Source: CAD feature listing. Evaluate the final solid. Frame: model axes, mm. Face numbers are marked on the shaded views. A direction names the side the tool comes from. Give positions to 0.01 mm unless a question says otherwise; leave off trailing zeros. Loops run counter-clockwise (first coordinate to the right, second up) from the corner with the lowest first, then second, coordinate; pieces in that order, holes last. Notation, with made-up numbers: M -3.5,70.5 L 52.5,70.5 A34 cw 52.5,106.5 Z; hole C 14,47 d8. An arc over 180 degrees is marked long. Write item = value, one per line.
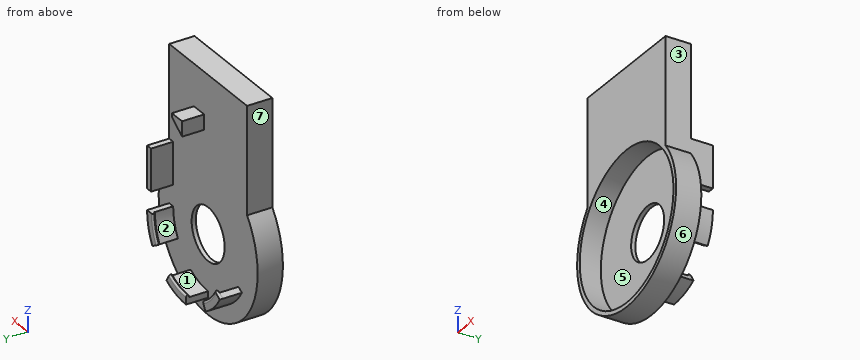
from build123d import *

# Parameters (mm, degrees)
SKETCH1_R           = 37.5
SKETCH1_R_2         = 35.5
BOSS_EXTRUDE1_DEPTH = 10
SKETCH2_R           = 37.5
SKETCH2_R_2         = 12.5
BOSS_EXTRUDE2_DEPTH = 2
BOSS_EXTRUDE3_DEPTH = 9
BOSS_EXTRUDE4_DEPTH = 1.5
FILLET1_R           = 1.27
SKETCH6_W           = 3
SKETCH6_H           = 10.5
BOSS_EXTRUDE5_DEPTH = 30
SKETCH7_W           = 3
SKETCH7_H           = 10
CUT_EXTRUDE1_DEPTH  = 10.5
BOSS_EXTRUDE6_DEPTH = 10.5
BOSS_EXTRUDE8_START = -12
BOSS_EXTRUDE8_DEPTH = 12


with BuildPart() as part:
    # Sketch1 → Boss-Extrude1 (new body)
    with BuildSketch(Plane(origin=(0, 0, 0), x_dir=(1, 0, 0), z_dir=(0, 1, 0))):
        with Locations(Location((0, 0, 0), (0, 0, 270))):
            Circle(SKETCH1_R)
        with Locations(Location((0, 0, 0), (0, 0, 270))):
            Circle(SKETCH1_R_2, mode=Mode.SUBTRACT)
    extrude(amount=BOSS_EXTRUDE1_DEPTH)

    # Sketch2 → Boss-Extrude2 (add)
    with BuildSketch(Plane(origin=(0, 10, 0), x_dir=(1, 0, 0), z_dir=(0, 1, 0))):
        with Locations(Location((0, 0, 0), (0, 0, 270))):
            Circle(SKETCH2_R)
        with Locations(Location((0, 0, 0), (0, 0, 270))):
            Circle(SKETCH2_R_2, mode=Mode.SUBTRACT)
    extrude(amount=BOSS_EXTRUDE2_DEPTH)

    # Sketch4 → Boss-Extrude3 (add)
    with BuildSketch(Plane(origin=(0, 12, 0), x_dir=(1, 0, 0), z_dir=(0, 1, 0))):
        with BuildLine():
            Line((13.25, 22.9496732), (14.75, 25.547749412))
            ThreePointArc((14.75, 25.547749412), (7.635161831, 28.494811876), (0, 29.5))
            Line((0, 29.5), (0, 26.5))
            ThreePointArc((0, 26.5), (6.858704695, 25.597034397), (13.25, 22.9496732))
        make_face()
        with BuildLine():
            ThreePointArc((26.5, 0), (25.597034397, 6.858704695), (22.9496732, 13.25))
            Line((22.9496732, 13.25), (25.547749412, 14.75))
            ThreePointArc((25.547749412, 14.75), (28.494811876, 7.635161831), (29.5, 0))
            Line((29.5, 0), (26.5, 0))
        make_face()
        with BuildLine():
            Line((-13.25, 22.9496732), (-14.75, 25.547749412))
            ThreePointArc((-14.75, 25.547749412), (-20.859650045, 20.859650045), (-25.547749412, 14.75))
            Line((-25.547749412, 14.75), (-22.9496732, 13.25))
            ThreePointArc((-22.9496732, 13.25), (-18.738329701, 18.738329701), (-13.25, 22.9496732))
        make_face()
    extrude(amount=BOSS_EXTRUDE3_DEPTH)

    # Sketch5 → Boss-Extrude4 (add)
    with BuildSketch(Plane(origin=(0, 21, 0), x_dir=(1, 0, 0), z_dir=(0, 1, 0))):
        with BuildLine():
            Line((-12.5, 21.650635095), (-14.75, 25.547749412))
            ThreePointArc((-14.75, 25.547749412), (-20.859650045, 20.859650045), (-25.547749412, 14.75))
            Line((-25.547749412, 14.75), (-21.650635095, 12.5))
            ThreePointArc((-21.650635095, 12.5), (-17.67766953, 17.67766953), (-12.5, 21.650635095))
        make_face()
        with BuildLine():
            ThreePointArc((0, 26.5), (6.858704695, 25.597034397), (13.25, 22.9496732))
            Line((13.25, 22.9496732), (14.75, 25.547749412))
            ThreePointArc((14.75, 25.547749412), (7.635161831, 28.494811876), (0, 29.5))
            Line((0, 29.5), (0, 26.5))
        make_face()
        with BuildLine():
            Line((0, 26.5), (0, 25))
            ThreePointArc((0, 25), (6.470476128, 24.148145657), (12.5, 21.650635095))
            Line((12.5, 21.650635095), (13.25, 22.9496732))
            ThreePointArc((13.25, 22.9496732), (6.858704695, 25.597034397), (0, 26.5))
        make_face()
        with BuildLine():
            Line((25, 0), (29.5, 0))
            ThreePointArc((29.5, 0), (28.494811876, 7.635161831), (25.547749412, 14.75))
            Line((25.547749412, 14.75), (21.650635095, 12.5))
            ThreePointArc((21.650635095, 12.5), (24.148145657, 6.470476128), (25, 0))
        make_face()
    extrude(amount=BOSS_EXTRUDE4_DEPTH)

    # Fillet1
    # the kernel refuses this fillet: 1.27 mm, written as the material it takes off along each edge
    with BuildSketch(Plane(origin=(0, 21, 0), x_dir=(0.795717852622937, 0, -0.605667482218702), z_dir=(-0.605667482218702, 0, -0.795717852622937))) as fillet1_piece_1:
        with BuildLine():
            CenterArc((25 + FILLET1_R, -FILLET1_R), FILLET1_R, 90, 90)
            Line((25 + FILLET1_R, 0), (25, 0))
            Line((25, 0), (25, -FILLET1_R))
        make_face()
    revolve(axis=Axis((0, 21, 0), (0, -1, 0)), revolution_arc=44.553777402, mode=Mode.SUBTRACT)
    with BuildSketch(Plane(origin=(0, 22.5, 0), x_dir=(0.795717852622937, 0, -0.605667482218702), z_dir=(-0.605667482218702, 0, -0.795717852622937))) as fillet1_piece_2:
        with BuildLine():
            CenterArc((25 + FILLET1_R, FILLET1_R), FILLET1_R, 180, 90)
            Line((25, FILLET1_R), (25, 0))
            Line((25, 0), (25 + FILLET1_R, 0))
        make_face()
    revolve(axis=Axis((0, 22.5, 0), (0, -1, 0)), revolution_arc=44.553777402, mode=Mode.SUBTRACT)
    with BuildSketch(Plane(origin=(0, 21, 0), x_dir=(-0.12666449953608933, 0, -0.9919456157256162), z_dir=(-0.9919456157256162, 0, 0.12666449953608933))) as fillet1_piece_3:
        with BuildLine():
            CenterArc((25 + FILLET1_R, -FILLET1_R), FILLET1_R, 90, 90)
            Line((25 + FILLET1_R, 0), (25, 0))
            Line((25, 0), (25, -FILLET1_R))
        make_face()
    revolve(axis=Axis((0, 21, 0), (0, -1, 0)), revolution_arc=44.553777402, mode=Mode.SUBTRACT)
    with BuildSketch(Plane(origin=(0, 22.5, 0), x_dir=(-0.12666449953608933, 0, -0.9919456157256162), z_dir=(-0.9919456157256162, 0, 0.12666449953608933))) as fillet1_piece_4:
        with BuildLine():
            CenterArc((25 + FILLET1_R, FILLET1_R), FILLET1_R, 180, 90)
            Line((25, FILLET1_R), (25, 0))
            Line((25, 0), (25 + FILLET1_R, 0))
        make_face()
    revolve(axis=Axis((0, 22.5, 0), (0, -1, 0)), revolution_arc=44.553777402, mode=Mode.SUBTRACT)
    with BuildSketch(Plane(origin=(0, 21, 0), x_dir=(-0.9223823521590265, 0, -0.386278133506909), z_dir=(-0.386278133506909, 0, 0.9223823521590265))) as fillet1_piece_5:
        with BuildLine():
            CenterArc((25 + FILLET1_R, -FILLET1_R), FILLET1_R, 90, 90)
            Line((25 + FILLET1_R, 0), (25, 0))
            Line((25, 0), (25, -FILLET1_R))
        make_face()
    revolve(axis=Axis((0, 21, 0), (0, -1, 0)), revolution_arc=44.553777402, mode=Mode.SUBTRACT)
    with BuildSketch(Plane(origin=(0, 22.5, 0), x_dir=(-0.9223823521590265, 0, -0.386278133506909), z_dir=(-0.386278133506909, 0, 0.9223823521590265))) as fillet1_piece_6:
        with BuildLine():
            CenterArc((25 + FILLET1_R, FILLET1_R), FILLET1_R, 180, 90)
            Line((25, FILLET1_R), (25, 0))
            Line((25, 0), (25 + FILLET1_R, 0))
        make_face()
    revolve(axis=Axis((0, 22.5, 0), (0, -1, 0)), revolution_arc=44.553777402, mode=Mode.SUBTRACT)

    # Sketch6 → Boss-Extrude5 (add)
    with BuildSketch(Plane.XY):
        with Locations((28, 17.25)):
            Rectangle(SKETCH6_W, SKETCH6_H)
    extrude(amount=BOSS_EXTRUDE5_DEPTH)

    # Sketch7 → Cut-Extrude1 (cut)
    with BuildSketch(Plane(origin=(0, 22.5, 0), x_dir=(1, 0, 0), z_dir=(0, 1, 0))):
        with Locations((28, -5)):
            Rectangle(SKETCH7_W, SKETCH7_H)
    extrude(amount=-CUT_EXTRUDE1_DEPTH, mode=Mode.SUBTRACT)



with BuildPart() as body_2:
    # Sketch8 → Boss-Extrude6 (new body)
    with BuildSketch(Plane(origin=(0, 12, 0), x_dir=(1, 0, 0), z_dir=(0, 1, 0))):
        Polygon((10.733196366, -52.441497251), (3, -47), (3, -54.148297887), (10.733196366, -54.148297887), align=None)
    extrude(amount=BOSS_EXTRUDE6_DEPTH)


with BuildPart() as part_1:
    add(part.part)

    add(body_2.part)  # Boss-Extrude8 merges body 2
    # Sketch9 → Boss-Extrude8 (add)
    with BuildSketch(Plane(origin=(0, 12, 0), x_dir=(1, 0, 0), z_dir=(0, 1, 0)).offset(BOSS_EXTRUDE8_START)):
        with BuildLine():
            Line((-26.911893282, -23.151673806), (-29.5, -23.151673806))
            Line((-29.5, -23.151673806), (-29.5, -73.951673806))
            Line((-29.5, -73.951673806), (29.5, -73.951673806))
            Line((29.5, -73.951673806), (29.5, -23.151673806))
            Line((29.5, -23.151673806), (26.911893282, -23.151673806))
            ThreePointArc((26.911893282, -23.151673806), (0, -35.5), (-26.911893282, -23.151673806))
        make_face()
    extrude(amount=BOSS_EXTRUDE8_DEPTH)


solid = part_1.part
1. Cut plane C-C, the plane y = 4.25. Return the cut outline in (x, z), then the cut area to 3 significant figures.
Derived:
outline = M -29.5,23.15 A37.5 ccw long 29.5,23.15 L 29.5,73.95 L -29.5,73.95 Z; hole C 0,0 d71
area = 2,870 mm²
2. Reachability of the marked faces 1, 2, 3 and 4 from +Z, -Z, +X, -X, +Y, -Y: full face, straight path, thin tool, end or side. Return the list, or none.
Derived:
face_1 = none
face_2 = +Z, -X
face_3 = +Z, +X, +Y
face_4 = -Y
3. Pull-direction query (Z, two-part tool) for the marked faces 5, 6 and 7; classes: +Z half, -Z half, draft (parallel to the pull), parting line (faces both ways), or undercut.
Derived:
face_5 = undercut
face_6 = parting line
face_7 = draft
4. Cut plane B-B, the plane z = 5. Return the cut outline in (x, y), then the cut area to 3 significant figures.
Derived:
outline = M -37.17,0 L -35.15,0 L -35.15,10 L -11.46,10 L -11.46,12 L -37.17,12 Z; M 11.46,10 L 35.15,10 L 35.15,0 L 37.17,0 L 37.17,12 L 11.46,12 Z
area = 143 mm²
5. First-contact query: pin 1 Ø1.1 at (x, z) = (5, -25) entering from -Y; pin 2 Ø7 at (y, z) = (6, 42) entering from +X; pin 3 Ø3.5 at (y, z) = (17.5, 51.5) entering from -X; pin 4 Ø22.5 at (x, z) = (0, 0) entering from +Y. Flat tips, straight axial feed; report the tip coordinate or a pass-through.
Derived:
pin_1 = 10
pin_2 = 29.5
pin_3 = 3
pin_4 = through
6. Cut plane D-D, the plane z = 33. Return the cut outline in (x, y), then the cut area to 3 significant figures.
Derived:
outline = M -29.5,0 L -13.09,0 L -13.09,10 L 13.09,10 L 13.09,0 L 29.5,0 L 29.5,12 L -29.5,12 Z
area = 446 mm²
7. Material intervals for probe 1 along X at (y, z) = (10.55, 0); probe 2 along X at (y, z) = (5.5, 0); probe 3 along Y at (x, z) = (-22, 45), sorted ascending. Write a range as from..to.
Derived:
probe_1 = -37.5..-12.5, 12.5..37.5
probe_2 = -37.5..-35.5, 35.5..37.5
probe_3 = 0..12
8. Cut plane A-A, the plane y = 17. Return the cut outline in (x, z).
Derived:
outline = M -25.55,-14.75 A29.5 ccw -14.75,-25.55 L -13.25,-22.95 A26.5 cw -22.95,-13.25 Z; M 0,-29.5 A29.5 ccw 14.75,-25.55 L 13.25,-22.95 A26.5 cw 0,-26.5 Z; M 3,47 L 10.73,52.44 L 10.73,54.15 L 3,54.15 Z; M 22.95,-13.25 L 25.55,-14.75 A29.5 ccw 29.5,0 L 26.5,0 A26.5 cw Z; M 26.5,10 L 29.5,10 L 29.5,30 L 26.5,30 Z
